from build123d import *

# Parameters (mm, degrees)
SKETCH_1_W          = 57.64
SKETCH_1_H          = 125
EXTRUDE_1_DEPTH     = 5
CUT_EXTRUDE_1_DEPTH = 2.5
SKETCH_3_W          = 57.64
SKETCH_3_H          = 30
CUT_EXTRUDE_2_DEPTH = 10


with BuildPart() as part:
    # 스케치1 → 보스-돌출1 (new body)
    with BuildSketch(Plane.XY):
        Rectangle(SKETCH_1_W, SKETCH_1_H)
    extrude(amount=EXTRUDE_1_DEPTH)

    # 스케치2 → 컷-돌출1 (cut)
    with BuildSketch(Plane.XY.offset(5)):
        with BuildLine():
            ThreePointArc((-5, 5.10170356), (0, 10.10170356), (5, 5.10170356))
            ThreePointArc((5, 5.10170356), (0, 0.10170356), (-5, 5.10170356))
        make_face()
    extrude(amount=-CUT_EXTRUDE_1_DEPTH, mode=Mode.SUBTRACT)

    # 스케치3 → 컷-돌출2 (cut)
    with BuildSketch(Plane.XY.offset(5)):
        with Locations((0, 47.5)):
            Rectangle(SKETCH_3_W, SKETCH_3_H)
    extrude(amount=-CUT_EXTRUDE_2_DEPTH, mode=Mode.SUBTRACT)


solid = part.part
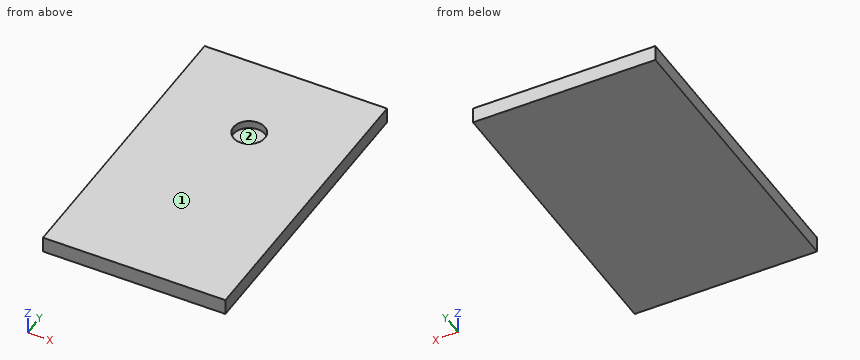
Work out the finished part from the listing and answer in its coordinate system (mm). Face numbers are marked on the shaded views. Round coordinates to 2 decimals unless told otherwise and drop trailing zeros. Loops run counter-clockwise (first coordinate to the right, second up) from the corner with the lowest first, then second, coordinate; pieces in that order, holes last. Notation, with made-up numbers: (42, 67) - (94, 67) arc R32 cw to (94, 95) - close; hole circle Ø4 at (80, 86). An arc over 180 degrees is marked (long way). Use one line per item in the form item = value. Start each with the question number.
(1) Find section B-B on y = 3.5. Determine the outline of the cut face in (x, z), and give its area (3 significant figures).
(2) Find section A-A on x = 0. Determine the outline of the cut face in (y, z).
(3) Determine the mould class of the marked faces 1 and 2 for opening direction X: +X half, -X half, draft (parallel to the pull), parting line (faces both ways), or undercut.
(4) A flat-ended cylindrical pin translates along its axis: P1, Ø3, axis at x = -2, y = 5, coming from the +Z side. Find the tip coordinate at first contact, or state that the pin passes through.
(5) Consider line 1 (Y direction, x = 0, z = 3.6). Determine where the line is inside the solid, lowest interval first.
Answer list:
q1.outline = (-28.82, 0) - (28.82, 0) - (28.82, 5) - (4.74, 5) - (4.74, 2.5) - (-4.74, 2.5) - (-4.74, 5) - (-28.82, 5) - close
q1.area = 265 mm^2
q2.outline = (-62.5, 0) - (32.5, 0) - (32.5, 5) - (10.1, 5) - (10.1, 2.5) - (0.1, 2.5) - (0.1, 5) - (-62.5, 5) - close
q3.face_1 = draft
q3.face_2 = undercut
q4.P1 = 2.5
q5.line_1 = -62.5 to 0.1, 10.1 to 32.5
